Geometry: final body of the model. Coordinates: model frame, mm. A direction names the side the tool comes from. Give positions to 0.01 mm unless a question says otherwise; leave off trailing zeros. Write each loop counter-clockwise with the first axis right and the second up, starting at its lowest first coordinate (ties: lowest second). Pieces come first, ordered by that corner, then holes.
Q1. Cut plane B-B on x = 98. Return the cut outline in (y, z), plus the area to 3 significant figures.
Q2. Cut plane A-A on y = -54. Return the cut outline in (x, z), plus the area to 3 significant figures.
Q3. Draft query along Y for faces 1 (the face through (209.222, 3.158, 1.503)), 2 (the face through (3.46, 11.29, 1.5)), 3 (the face through (204.395, -108.531, 1.503)), 4 (the face through (189.884, 30.332, 1.503)). Return one class per face: pulls with the +Y half, pulls with the -Y half, needs draft (parallel to the pull), parting line crosses it, or undercut.
Q4. Pin query (flat end, axial travel): pin 1 (1.5 mm diameter, centred on y = 3.5, z = 1, fed in from -X). Return the tip coordinate at first contact, or that it passes through.
Q5. Cut plane D-D on z = 1.55. Count the separate pieces of the cut face and the enclosed holes in it, plus the area to 3 significant figures.
Q6. Reachability of faces 5 (the face through (20.187, -108.531, 1.503)), 6 (the face through (16.959, -45.893, 1.503)) from +Z, -Z, +X, -X, +Y, -Y: full face, straight path, thin tool, end or side. Return the list, or none.
Q7. Cut plane C-C on y = -150.5. Return the cut outline in (x, z).
Q8. Line query: L1, parallel to Y at x = 122.5, z = 2.15; L2, parallel to Y at x = 179, z = 1.55; L3, parallel to X at y = 5.5, z = 1.1. Output: solid intervals per line, ascending.
Autodesk Inventor part; units mm, degrees
ref_plane "YZ Plane" through (0, 0, 0) normal (1, 0, 0) x (0, 1, 0)
ref_plane "XZ Plane" through (0, 0, 0) normal (0, 1, 0) x (-1, 0, 0)
ref_plane "XY Plane" through (0, 0, 0) normal (0, 0, 1) x (1, 0, 0)
sketch "Base" plane through (0, 0, 0) normal (0, 0, 1) x (1, 0, 0)
  circle A0 centre (12.187819, 3.297819) radius 3.175
  circle A1 centre (-5.772693, -14.662693) radius 3.175
  circle A2 centre (212.394424, 3.297819) radius 3.175
  circle A3 centre (230.354936, -14.662693) radius 3.175
  arc A4 (-21.168075, -17.047312) -> (9.622688, 23.64295) centre (-130.364106, 97.577494) ccw construction
  arc A5 (214.959555, 23.64295) -> (245.750318, -17.047312) centre (354.946349, 97.577494) ccw construction
  line L0 (26.243247, 41.397819) -> (-19.976862, -19.682458)
  line L1 (12.187819, 3.297819) -> (212.394424, 3.297819) construction
  line L2 (112.291121, 41.397819) -> (112.291121, -199.902181) construction
  line L3 (26.243247, 41.397819) -> (112.291121, 41.397819)
  line L4 (-19.976862, -19.682458) -> (61.491121, -199.902181)
  line L5 (61.491121, -199.902181) -> (112.291121, -199.902181)
  line L6 (9.622688, 23.64295) -> (-21.168075, -17.047312) construction
  line L7 (-19.976862, -19.682458) -> (-21.168075, -17.047312) construction
  line L8 (62.346745, -145.552947) -> (162.235762, -145.552947) construction
  line L9 (89.431121, 18.537819) -> (89.431121, -177.042181) construction
  line L10 (89.431121, -177.042181) -> (76.244498, -177.042181)
  line L11 (76.244498, -177.042181) -> (6.449214, -22.644267)
  line L12 (6.449214, -22.644267) -> (37.612145, 18.537819)
  line L13 (37.612145, 18.537819) -> (89.431121, 18.537819)
  line L14 (89.431121, 18.537819) -> (112.291121, 18.537819)
  line L15 (89.431121, -177.042181) -> (112.291121, -177.042181)
  line L16 (198.338996, 41.397819) -> (244.559105, -19.682458)
  line L17 (198.338996, 41.397819) -> (112.291121, 41.397819)
  line L18 (244.559105, -19.682458) -> (163.091121, -199.902181)
  line L19 (163.091121, -199.902181) -> (112.291121, -199.902181)
  line L20 (135.151121, -177.042181) -> (148.337745, -177.042181)
  line L21 (148.337745, -177.042181) -> (218.133029, -22.644267)
  line L22 (218.133029, -22.644267) -> (186.970097, 18.537819)
  line L23 (186.970097, 18.537819) -> (135.151121, 18.537819)
  line L24 (135.151121, 18.537819) -> (112.291121, 18.537819)
  line L25 (135.151121, -177.042181) -> (112.291121, -177.042181)
  point P0 (0, 0)
  point P1 (112.291121, 3.297819)
extrude "Plate1" add sketch "Base" along normal blind 3.048
sketch "Sketch2" plane through (0, 0, 3.048) normal (0, 0, 1) x (1, 0, 0)
  circle A0 centre (104.291121, -48.262182) radius 2.05
  circle A1 centre (104.291121, -32.262181) radius 2.05
  circle A2 centre (120.291122, -32.262181) radius 2.05
  circle A3 centre (120.291122, -48.262182) radius 2.05
  line L0 (120.291122, -32.262181) -> (104.291121, -32.262181) construction
  line L1 (104.291121, -32.262181) -> (104.291121, -48.262182) construction
  line L2 (104.291121, -48.262182) -> (120.291122, -48.262182) construction
  line L3 (120.291122, -48.262182) -> (120.291122, -32.262181) construction
  line L4 (186.970097, 18.537819) -> (37.612145, 18.537819)
  line L5 (148.337745, -177.042181) -> (76.244498, -177.042181)
  line L6 (112.291121, 18.537819) -> (112.291121, -177.042181) construction
  line L7 (76.244498, -177.042181) -> (148.337745, -177.042181)
  line L8 (122.451121, 18.537819) -> (122.451121, -19.562181)
  line L9 (122.451121, -19.562181) -> (139.767673, -42.446156)
  line L10 (139.767673, -42.446156) -> (197.403821, -68.500466)
  line L11 (218.133029, -22.644267) -> (148.337745, -177.042181)
  line L12 (189.033686, -87.016493) -> (131.397539, -60.962182)
  line L13 (131.397539, -60.962182) -> (112.291121, -60.962182)
  line L14 (218.133029, -22.644267) -> (186.970097, 18.537819)
  line L15 (148.337745, -177.042181) -> (218.133029, -22.644267)
  line L16 (122.451121, -19.562181) -> (112.291121, -19.562181) construction
  line L17 (139.767673, -42.446156) -> (131.397539, -60.962182) construction
  line L18 (102.131121, 18.537819) -> (102.131121, -19.562181)
  line L19 (102.131121, -19.562181) -> (84.81457, -42.446156)
  line L20 (84.81457, -42.446156) -> (27.178422, -68.500466)
  line L21 (35.548557, -87.016493) -> (93.184704, -60.962182)
  line L22 (93.184704, -60.962182) -> (112.291121, -60.962182)
  line L23 (122.451121, 18.537819) -> (102.131121, 18.537819)
  line L24 (197.403821, -68.500466) -> (189.033686, -87.016493)
  line L25 (27.178422, -68.500466) -> (35.548557, -87.016493)
  line L26 (76.244498, -177.042181) -> (6.449214, -22.644267)
  point P0 (0, 0)
  point P1 (112.291121, -32.262181)
  dimension "d8" = 16
  dimension "d9" = 16
  dimension "d10" = 50.8
  dimension "d11" = 10.16
  dimension "d12" = 20.32
  dimension "d13" = 12.7
  dimension "d14" = 12.7
sheet face with bend "Face2" sketch "Sketch2" thickness 3.048 toward (0, 0, -1) bend radius 3.048 contours L8 L9 L10 L11 L12 L13 L22 L21 L25 L20 L19 L18 L4
bend "Bend1"
sketch "Sketch3" plane through (0, 0, 3.048) normal (0, 0, 1) x (1, 0, 0)
  circle A0 centre (31.927696, 29.967819) radius 2.794
  line L0 (26.243247, 41.397819) -> (-19.976862, -19.682458)
  line L1 (6.449214, -22.644267) -> (37.612145, 18.537819)
  line L2 (26.243247, 41.397819) -> (37.612145, 18.537819) construction
  line L3 (186.970097, 18.537819) -> (218.133029, -22.644267)
  line L4 (244.559105, -19.682458) -> (198.338996, 41.397819)
  line L5 (186.970097, 18.537819) -> (198.338996, 41.397819) construction
  circle A1 centre (192.654547, 29.967819) radius 2.794
  line L6 (27.178422, -68.500466) -> (6.449214, -22.644267)
  line L7 (27.178422, -68.500466) -> (35.548557, -87.016493) construction
  line L8 (31.36349, -77.75848) -> (10.53296, -87.174881) construction
  line L9 (61.491121, -199.902181) -> (-19.976862, -19.682458)
  circle A2 centre (20.948225, -82.466681) radius 2.794
  line L10 (26.243247, 41.397819) -> (198.338996, 41.397819)
  line L11 (112.291121, 41.397819) -> (112.291121, -60.962182) construction
  line L12 (93.184704, -60.962182) -> (131.397539, -60.962182)
  circle A3 centre (203.634018, -82.466681) radius 2.794
  point P0 (0, 0)
  dimension "d20" = 5.588
  dimension "d21" = 5.588
hole "Hole1" at (31.927696, 29.967819, 3.048) at (192.654547, 29.967819, 3.048) at (20.948225, -82.466681, 3.048) at (203.634018, -82.466681, 3.048) direction (0, 0, -1) diameter 5.588 end through all
equation "\"d12\" = 2 * d11"
equation "\"d27\" = Thickness"
equation "\"d7\" = Thickness"
equation "\"d15\" = BendRadius"
equation "\"d16\" = BendReliefWidth"
equation "\"d18\" = MinimumRemnant"
equation "\"d17\" = BendReliefDepth"
equation "\"d19\" = TransitionRadius"
equation "\"BendRadius\" = Thickness"
equation "\"BendReliefWidth\" = Thickness"
equation "\"BendReliefDepth\" = 0.5 * Thickness"
equation "\"CornerReliefSize\" = 4 * Thickness"
equation "\"MinimumRemnant\" = 2 * Thickness"
equation "\"TransitionRadius\" = BendRadius"
equation "\"JacobiRadiusSize\" = BendRadius"
equation "\"GapSize\" = Thickness"
properties part number "ChestMount"
Data:
1. outline: (-199.9, 0) - (-177.04, 0) - (-177.04, 3.05) - (-199.9, 3.05) - close; (-60.96, 0) - (-25.02, 0) - (-25.02, 3.05) - (-60.96, 3.05) - close; (18.54, 0) - (41.4, 0) - (41.4, 3.05) - (18.54, 3.05) - close
1. area: 249 mm2
2. outline: (-4.46, 0) - (20.62, 0) - (20.62, 3.05) - (-4.46, 3.05) - close; (59.26, 0) - (165.33, 0) - (165.33, 3.05) - (59.26, 3.05) - close; (203.96, 0) - (229.05, 0) - (229.05, 3.05) - (203.96, 3.05) - close
2. area: 476 mm2
3. face 1: undercut
3. face 2: pulls with the +Y half
3. face 3: pulls with the -Y half
3. face 4: undercut
4. pin 1: stops at x = -3
5. separate pieces: 1
5. enclosed holes: 15
5. area: 21,800 mm2
6. face 5: +Z, -Z, -X, -Y
6. face 6: +Z, -Z
7. outline: (39.16, 0) - (64.25, 0) - (64.25, 3.05) - (39.16, 3.05) - close; (160.34, 0) - (185.42, 0) - (185.42, 3.05) - (160.34, 3.05) - close
8. L1: y = -199.9 to -177.04, -60.96 to -19.63, 18.54 to 41.4
8. L2: y = -164.71 to -109.21, -82.48 to -60.18, 18.54 to 41.4
8. L3: x = -0.92 to 9.9, 14.47 to 27.75, 102.13 to 122.45, 196.84 to 210.11, 214.68 to 225.5
